```python
from build123d import *

# Parameters (mm, degrees)
BOSS_EXTRUDE1_DEPTH = 16
SKETCH2_R           = 8.75
BOSS_EXTRUDE2_DEPTH = 1
BOSS_EXTRUDE3_START = 6
SKETCH3_R           = 8.75
BOSS_EXTRUDE3_DEPTH = 6
SKETCH4_R           = 4
CUT_EXTRUDE1_DEPTH  = 27.117522853
SKETCH5_R           = 2
CUT_EXTRUDE2_DEPTH  = 22.026768653
CIRPATTERN1_COUNT   = 2
CIRPATTERN1_ANGLE   = 90


with BuildPart() as part:
    # Sketch1 → Boss-Extrude1 (new body)
    with BuildSketch(Plane.XY):
        with BuildLine():
            ThreePointArc((0, 5.325), (1.029470644, 5.724915472), (1.519005236, 6.7149145))
            ThreePointArc((1.519005236, 6.7149145), (1.704817188, 7.031923192), (2.067709649, 7.089626352))
            ThreePointArc((2.067709649, 7.089626352), (2.282090503, 7.023552373), (2.494365569, 6.95099744))
            ThreePointArc((2.494365569, 6.95099744), (2.75403467, 6.691011766), (2.718026663, 6.325328822))
            ThreePointArc((2.718026663, 6.325328822), (2.53216164, 5.236661571), (3.129956468, 4.308015495))
            ThreePointArc((3.129956468, 4.308015495), (4.197880131, 4.026446247), (5.175828764, 4.53963107))
            ThreePointArc((5.175828764, 4.53963107), (5.512486825, 4.686878964), (5.839990059, 4.520258965))
            ThreePointArc((5.839990059, 4.520258965), (5.974590503, 4.340794088), (6.103677919, 4.157323762))
            ThreePointArc((6.103677919, 4.157323762), (6.16093889, 3.794361265), (5.916864759, 3.519682524))
            ThreePointArc((5.916864759, 3.519682524), (5.126594241, 2.748180936), (5.064375949, 1.645515495))
            ThreePointArc((5.064375949, 1.645515495), (5.762842089, 0.790011408), (6.855661624, 0.630362868))
            ThreePointArc((6.855661624, 0.630362868), (7.214573857, 0.551606273), (7.381592761, 0.224306291))
            ThreePointArc((7.381592761, 0.224306291), (7.385, 0), (7.381592761, -0.224306291))
            ThreePointArc((7.381592761, -0.224306291), (7.214573857, -0.551606273), (6.855661624, -0.630362868))
            ThreePointArc((6.855661624, -0.630362868), (5.762842089, -0.790011408), (5.064375949, -1.645515495))
            ThreePointArc((5.064375949, -1.645515495), (5.126594241, -2.748180936), (5.916864759, -3.519682524))
            ThreePointArc((5.916864759, -3.519682524), (6.16093889, -3.794361265), (6.103677919, -4.157323762))
            ThreePointArc((6.103677919, -4.157323762), (5.974590503, -4.340794088), (5.839990059, -4.520258965))
            ThreePointArc((5.839990059, -4.520258965), (5.512486825, -4.686878964), (5.175828764, -4.53963107))
            ThreePointArc((5.175828764, -4.53963107), (4.197880131, -4.026446247), (3.129956468, -4.308015495))
            ThreePointArc((3.129956468, -4.308015495), (2.532161639, -5.236661571), (2.718026663, -6.325328822))
            ThreePointArc((2.718026663, -6.325328822), (2.75403467, -6.691011766), (2.494365569, -6.95099744))
            ThreePointArc((2.494365569, -6.95099744), (2.282090503, -7.023552373), (2.067709649, -7.089626352))
            ThreePointArc((2.067709649, -7.089626352), (1.704817188, -7.031923192), (1.519005236, -6.7149145))
            ThreePointArc((1.519005236, -6.7149145), (1.029470644, -5.724915472), (0, -5.325))
            ThreePointArc((0, -5.325), (-1.029470644, -5.724915472), (-1.519005236, -6.7149145))
            ThreePointArc((-1.519005236, -6.7149145), (-1.704817188, -7.031923192), (-2.067709649, -7.089626352))
            ThreePointArc((-2.067709649, -7.089626352), (-2.282090503, -7.023552373), (-2.494365569, -6.95099744))
            ThreePointArc((-2.494365569, -6.95099744), (-2.75403467, -6.691011766), (-2.718026663, -6.325328822))
            ThreePointArc((-2.718026663, -6.325328822), (-2.53216164, -5.236661571), (-3.129956468, -4.308015495))
            ThreePointArc((-3.129956468, -4.308015495), (-4.197880131, -4.026446247), (-5.175828764, -4.53963107))
            ThreePointArc((-5.175828764, -4.53963107), (-5.512486825, -4.686878964), (-5.839990059, -4.520258965))
            ThreePointArc((-5.839990059, -4.520258965), (-5.974590503, -4.340794088), (-6.103677919, -4.157323762))
            ThreePointArc((-6.103677919, -4.157323762), (-6.16093889, -3.794361265), (-5.916864759, -3.519682524))
            ThreePointArc((-5.916864759, -3.519682524), (-5.126594241, -2.748180936), (-5.064375949, -1.645515495))
            ThreePointArc((-5.064375949, -1.645515495), (-5.762842089, -0.790011408), (-6.855661624, -0.630362868))
            ThreePointArc((-6.855661624, -0.630362868), (-7.214573857, -0.551606273), (-7.381592761, -0.224306291))
            ThreePointArc((-7.381592761, -0.224306291), (-7.385, 0), (-7.381592761, 0.224306291))
            ThreePointArc((-7.381592761, 0.224306291), (-7.214573857, 0.551606273), (-6.855661624, 0.630362868))
            ThreePointArc((-6.855661624, 0.630362868), (-5.762842089, 0.790011408), (-5.064375949, 1.645515495))
            ThreePointArc((-5.064375949, 1.645515495), (-5.126594241, 2.748180936), (-5.916864759, 3.519682524))
            ThreePointArc((-5.916864759, 3.519682524), (-6.16093889, 3.794361265), (-6.103677919, 4.157323762))
            ThreePointArc((-6.103677919, 4.157323762), (-5.974590503, 4.340794088), (-5.839990059, 4.520258965))
            ThreePointArc((-5.839990059, 4.520258965), (-5.512486825, 4.686878964), (-5.175828764, 4.53963107))
            ThreePointArc((-5.175828764, 4.53963107), (-4.197880131, 4.026446247), (-3.129956468, 4.308015495))
            ThreePointArc((-3.129956468, 4.308015495), (-2.532161639, 5.236661571), (-2.718026663, 6.325328822))
            ThreePointArc((-2.718026663, 6.325328822), (-2.75403467, 6.691011766), (-2.494365569, 6.95099744))
            ThreePointArc((-2.494365569, 6.95099744), (-2.282090503, 7.023552373), (-2.067709649, 7.089626352))
            ThreePointArc((-2.067709649, 7.089626352), (-1.704817188, 7.031923192), (-1.519005236, 6.7149145))
            ThreePointArc((-1.519005236, 6.7149145), (-1.029470644, 5.724915472), (0, 5.325))
        make_face()
    extrude(amount=BOSS_EXTRUDE1_DEPTH)

    # Sketch2 → Boss-Extrude2 (add)
    with BuildSketch(Plane.XY.offset(16)):
        Circle(SKETCH2_R)
    extrude(amount=BOSS_EXTRUDE2_DEPTH)

    # Sketch3 → Boss-Extrude3 (add)
    with BuildSketch(Plane(origin=(0, 0, 0), x_dir=(-1, 0, 0), z_dir=(0, 0, -1)).offset(BOSS_EXTRUDE3_START)):
        with Locations(Location((0, 0, 0), (0, 0, 180))):
            Circle(SKETCH3_R)
    extrude(amount=-BOSS_EXTRUDE3_DEPTH)

    # Sketch4 → Cut-Extrude1 (cut, through all)
    with BuildSketch(Plane(origin=(0, 0, -6), x_dir=(-1, 0, 0), z_dir=(0, 0, -1))):
        Circle(SKETCH4_R)
    extrude(amount=-CUT_EXTRUDE1_DEPTH, mode=Mode.SUBTRACT)

    # Sketch5 → Cut-Extrude2 (cut, through all)
    with BuildSketch(Plane(origin=(0, 0, 0), x_dir=(1, 0, 0), z_dir=(0, 1, 0))):
        with Locations(Location((0, 3, 0), (0, 0, 270))):
            Circle(SKETCH5_R)
    cut_extrude2 = extrude(amount=-CUT_EXTRUDE2_DEPTH, mode=Mode.SUBTRACT)

    # CirPattern1: Cut-Extrude2 ×2 about axis
    cirpattern1_axis = Axis((0, 0, 16), (0, 0, 1))
    for i in range(1, CIRPATTERN1_COUNT):
        add(cut_extrude2.rotate(cirpattern1_axis, i * CIRPATTERN1_ANGLE / (CIRPATTERN1_COUNT - 1)), mode=Mode.SUBTRACT)


solid = part.part
```
Here's how the part is built. I have some questions about the finished solid (model axes, mm). A direction names the side the tool comes from. Coordinates: 2 decimals unless noted, no trailing zeros. Order: outer loops, then holes, each group sorted by start corner. A loop starts at its lowest first (then second) coordinate and runs counter-clockwise, first axis right, second up.
1) Will these pins go through, and if not, where does the flat tip stop? pin 1 (2 mm diameter, centred on x = 1.5, z = -2.5, fed in from -Y); pin 2 (4 mm diameter, centred on x = -4.5, z = 7.5, fed in from +Y); pin 3 (8 mm diameter, centred on y = -1, z = -1, fed in from -X); pin 4 (2 mm diameter, centred on x = 0, y = 2.5, fed in from -Z).
2) Imagine slicing it at A-A on z = -3. List the corners of the cut face in (x, y) for me, and give its area (3 significant figures).
3) We'd pull the mould along Z, two halves only. Please class faces 4 (the face through (4, 2, -6)), 5 (the face through (0, -6, 16)), 6 (the face through (6.07, -0.766, -1.153)), 7 (the face through (4, -2, 17)): +Z half, -Z half, draft (parallel to the pull), parting line (faces both ways), or undercut.
4) Which directions (+Z, -Z, +X, -X, +Y, -Y) give clear straight access to the entire face, cutting with the end or side of a thin tool? Please do faces 1 (the face through (-1.9, 8.54, -3.04)), 2 (the face through (-0.766, -6.073, -1.153)), 3 (the face through (0, 6, 0)).
5) I need wall thicknesses on line 1 (Z direction, x = 0, y = -6.35); line 2 (Z direction, x = -6.25, y = -5.5); line 3 (Y direction, x = -6, z = 3). Which ranges of each line are inside material? Lowest first, please.
Response values:
1. pin 1: stops at y = -8.65
1. pin 2: stops at y = 6.95
1. pin 3: stops at x = -8.75
1. pin 4: passes through
2. outline: (-2, -8.52) - (-2, -3.46) arc R4 cw (long way) to (3.46, 2) - (8.52, 2) arc R8.75 ccw (long way) to start; (2, -8.52) arc R8.75 ccw to (8.52, -2) - (3.46, -2) arc R4 cw to (2, -3.46) - close
2. area: 151 mm2
3. face 4: -Z half
3. face 5: undercut
3. face 6: undercut
3. face 7: +Z half
4. face 1: +Z, -Z
4. face 2: -Y
4. face 3: none
5. line 1: z = -6 to -5, -1 to 0, 16 to 17
5. line 2: z = -6 to 0, 16 to 17
5. line 3: y = -4.31 to -3.57, -0.68 to 0.68, 3.57 to 4.31
